from build123d import *

# Parameters (mm, degrees)
F0_R     = 7.925
F1_DEPTH = 55
F3_SIZE2 = 0.349101
F3_SIZE  = 20
F2_R     = 2
F4_DEPTH = 40


with BuildPart() as f1:
    # F0 (on Top) → F1 (new body)
    with BuildSketch(Plane.XY):
        Circle(F0_R)
    extrude(amount=F1_DEPTH)

    # F3
    f3_edges = [f1.edges().sort_by_distance(p)[0] for p in [
        (-7.925, 0, 0),
    ]]
    chamfer(f3_edges, length=F3_SIZE, length2=F3_SIZE2)

    # F2 (on face) → F4 (cut)
    with BuildSketch(Plane.XY.offset(55)):
        Circle(F2_R)
    extrude(amount=-F4_DEPTH, mode=Mode.SUBTRACT)


solid = f1.part
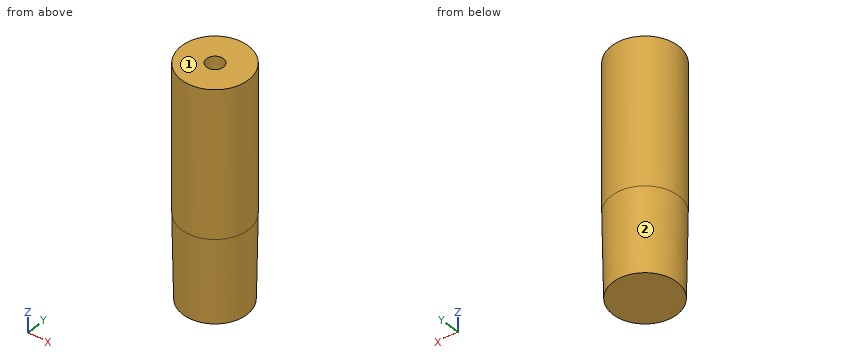
Verification items for the finished model (mm, model axes). Face numbers are marked on the shaded views. A direction names the side the tool comes from. Coordinates: 2 decimals unless noted, no trailing zeros. Loops run counter-clockwise (first coordinate to the right, second up) from the corner with the lowest first, then second, coordinate; pieces in that order, holes last. Notation, with made-up numbers: (49.25, 64.5) -> (66.25, 64.5) arc R17 cw to (66.25, 90.5) -> close; hole circle Ø1 at (10.5, 55). An arc over 180 degrees is marked (long way). Answer as a JSON object with one key per item and string values. Group by question number.
Item 1: Tool access check on the marked faces 1 and 2. Record the directions out of +Z, -Z, +X, -X, +Y, -Y that give a thin tool (end or side, any length) a straight path to the whole face; none if there is none.
Item 2: Depth check by flat-ended pin: pin 1 (2 mm diameter, centred on x = 0, y = 0, fed in from +Z); pin 2 (3 mm diameter, centred on x = 1.5, z = 15.5, fed in from +Y). Enter the tip coordinate at first touch or a pass-through.
Item 3: Scan lines: probe 1 along Y at (x, z) = (0, 38) (3 decimals); probe 2 along Z at (x, y) = (-1.5, -1.25); probe 3 along X at (y, z) = (2.75, 44). Record each from-to range of solid material in increasing order.
Item 4: Sectioned sample at A-A on z = 48.5. Record the boundary of the cut face in (x, y) (3 decimals).
Item 5: Sectioned sample at B-B on z = 12. Record the boundary of the cut face in (x, y).
Evaluation:
{
 "1": {"face 1": "+Z, +X, -X, +Y, -Y", "face 2": "-Z"},
 "2": {"pin 1": "stops at z = 15", "pin 2": "stops at y = 7.86"},
 "3": {"probe 1": "y = -7.925 to -2, 2 to 7.925", "probe 2": "z = 0 to 15", "probe 3": "x = -7.43 to 7.43"},
 "4": {"outline": "circle Ø15.85 at (0, 0); hole circle Ø4 at (0, 0)"},
 "5": {"outline": "circle Ø15.57 at (0, 0)"}
}
